Read the model definition and answer for the solid it produces. Units are mm, in the model's axes. Face numbers are marked on the shaded views. Coordinates: 2 decimals unless noted, no trailing zeros. Write each loop counter-clockwise with the first axis right and the second up, starting at its lowest first coordinate (ties: lowest second). Pieces come first, ordered by that corner, then holes.
(1) The part is cut by section D-D, the plane y = 71.5. Determine the outline of the cut face in (x, z).
(2) The part is cut by section A-A, the plane z = 6.5. Determine the outline of the cut face in (x, y), and give its area (3 significant figures).
(3) Straight lines are drawn through the part: line 1 along X through (y, z) = (116, 31.5); line 2 along Y through (x, z) = (4, 33.25); line 3 along X through (y, z) = (36, 23.5). For each, find the intervals that lie inside material, in ascending order.
(4) The part is cut by section B-B, the plane x = 58. Determine the outline of the cut face in (y, z).
(5) Given pin 1 (1.5 mm diameter, centred on x = 81.5, y = 110, fed in from +Z), flat-ended and moving along its own axis, determine where the tip first touches the part or whether it passes through.
(6) Determine the mould class of the marked faces 1, 2, 3 and 4 for opening direction X: pulls with the +X half, pulls with the -X half, needs draft (parallel to the pull), parting line crosses it, or undercut.
(7) The part is cut by section C-C, the plane x = 41. Determine the outline of the cut face in (y, z), and give its area (3 significant figures).
```python
from build123d import *

# Parameters (mm, degrees)
F0_W      = 88
F0_H      = 120
F1_DEPTH  = 3
F2_W      = 88
F2_H      = 120
F3_DEPTH  = 40
F5_DEPTH  = 3
F7_DEPTH  = 3
F8_R      = 0.5
F10_DEPTH = 20
F13_D     = 2.5
F13_DEPTH = 10
F13_TIP   = 0.7510757738
F15_DEPTH = 43
F17_DEPTH = 43
F18_W     = 10
F18_H     = 0.75
F19_DEPTH = 3
F21_D     = 2.5
F21_DEPTH = 25
F21_TIP   = 0.7510757738
F22_W     = 18
F22_H     = 3
F23_DEPTH = 3
F24_W     = 2
F24_H     = 12
F25_DEPTH = 3


with BuildPart() as f1:
    # F0 (on Top) → F1 (new body)
    with BuildSketch(Plane.XY):
        with Locations((44, 60)):
            Rectangle(F0_W, F0_H)
    extrude(amount=F1_DEPTH)

    # F2 (on face) → F3 (join)
    with BuildSketch(Plane.XY.offset(3)):
        with Locations((44, 60)):
            Rectangle(F2_W, F2_H)
        with BuildLine():
            ThreePointArc((3, 113.1715728753), (6.1213203436, 113.8786796564), (6.8284271247, 117))
            Line((6.8284271247, 117), (81.1715728753, 117))
            ThreePointArc((81.1715728753, 117), (81.8786796564, 113.8786796564), (85, 113.1715728753))
            Line((85, 113.1715728753), (85, 6.8284271247))
            ThreePointArc((85, 6.8284271247), (81.8786796564, 6.1213203436), (81.1715728753, 3))
            Line((81.1715728753, 3), (6.8284271247, 3))
            ThreePointArc((6.8284271247, 3), (6.1213203436, 6.1213203436), (3, 6.8284271247))
            Line((3, 6.8284271247), (3, 113.1715728753))
        make_face(mode=Mode.SUBTRACT)
    extrude(amount=F3_DEPTH)

    # F4 (on face) → F5 (cut, through all)
    with BuildSketch(Plane(origin=(0, 0, 0), x_dir=(0, -1, 0), z_dir=(-1, 0, 0))):
        with BuildLine():
            Line((-61.5, 38.8388347648), (-65.9194173824, 34.4194173824))
            ThreePointArc((-65.9194173824, 34.4194173824), (-61.5, 23.75), (-57.0805826176, 34.4194173824))
            Line((-57.0805826176, 34.4194173824), (-61.5, 38.8388347648))
        make_face()
        with BuildLine():
            Line((-39.0805826176, 34.4194173824), (-43.5, 38.8388347648))
            Line((-43.5, 38.8388347648), (-47.9194173824, 34.4194173824))
            ThreePointArc((-47.9194173824, 34.4194173824), (-43.5, 23.75), (-39.0805826176, 34.4194173824))
        make_face()
        with BuildLine():
            Line((-21.0805826176, 34.4194173824), (-25.5, 38.8388347648))
            Line((-25.5, 38.8388347648), (-29.9194173824, 34.4194173824))
            ThreePointArc((-29.9194173824, 34.4194173824), (-25.5, 23.75), (-21.0805826176, 34.4194173824))
        make_face()
    extrude(amount=-F5_DEPTH, mode=Mode.SUBTRACT)

    # F6 (on face) → F7 (cut, through all)
    with BuildSketch(Plane(origin=(0, 120, 0), x_dir=(-1, 0, 0), z_dir=(0, 1, 0))):
        with BuildLine():
            Line((-54.9344657888, 16.95), (-61.0655342112, 16.95))
            ThreePointArc((-61.0655342112, 16.95), (-58, 8), (-54.9344657888, 16.95))
        make_face()
    extrude(amount=-F7_DEPTH, mode=Mode.SUBTRACT)

    # F8
    f8_edges = [f1.edges().sort_by_distance(p)[0] for p in [
        (0, 60, 0),
        (44, 0, 0),
        (0, 0, 21.5),
        (0, 120, 21.5),
        (88, 0, 21.5),
        (88, 60, 0),
        (44, 120, 0),
        (88, 120, 21.5),
    ]]
    fillet(f8_edges, radius=F8_R)

    # F9 (on face) → F10 (join)
    with BuildSketch(Plane.XY.offset(3)):
        with BuildLine():
            Line((6.5, 84), (3, 84))
            Line((3, 84), (3, 74))
            Line((3, 74), (6.5, 74))
            ThreePointArc((6.5, 74), (11.5, 79), (6.5, 84))
        make_face()
        with BuildLine():
            Line((3, 105), (6.5, 105))
            ThreePointArc((6.5, 105), (10.0355339059, 106.4644660941), (11.5, 110))
            Line((11.5, 110), (11.5, 117))
            Line((11.5, 117), (6.8284271247, 117))
            ThreePointArc((6.8284271247, 117), (6.1213203436, 113.8786796564), (3, 113.1715728753))
            Line((3, 113.1715728753), (3, 105))
        make_face()
        with BuildLine():
            Line((81.1715728753, 117), (76.5, 117))
            Line((76.5, 117), (76.5, 110))
            ThreePointArc((76.5, 110), (77.9644660941, 106.4644660941), (81.5, 105))
            Line((81.5, 105), (85, 105))
            Line((85, 105), (85, 113.1715728753))
            ThreePointArc((85, 113.1715728753), (81.8786796564, 113.8786796564), (81.1715728753, 117))
        make_face()
        with BuildLine():
            Line((85, 74), (85, 84))
            Line((85, 84), (81.5, 84))
            ThreePointArc((81.5, 84), (76.5, 79), (81.5, 74))
            Line((81.5, 74), (85, 74))
        make_face()
    extrude(amount=F10_DEPTH)

    # F13
    with Locations(Plane.XY.offset(23)):
        with Locations((6.5, 110), (6.5, 79), (81.5, 79), (81.5, 110)):
            Hole(F13_D / 2, depth=F13_DEPTH)
            with Locations((0, 0, -(F13_DEPTH + F13_TIP / 2))):  # 118° drill point
                Cone(0, F13_D / 2, F13_TIP, mode=Mode.SUBTRACT)

    # F14 (on face) → F15 (cut, through all)
    with BuildSketch(Plane.XZ.offset(-74)):
        Polygon((76.5, 3), (85, 3), (85, 9), (76.5, 21.1392580573), align=None)
    extrude(amount=-F15_DEPTH, mode=Mode.SUBTRACT)

    # F16 (on face) → F17 (cut, through all)
    with BuildSketch(Plane.XZ.offset(-74)):
        Polygon((3, 9), (3, 3), (11.5, 3), (11.5, 21.1392580573), align=None)
    extrude(amount=-F17_DEPTH, mode=Mode.SUBTRACT)

    # F18 (on face) → F19 (cut, through all)
    with BuildSketch(Plane.XY.offset(3)):
        with Locations((80, 7.875)):
            Rectangle(F18_W, F18_H)
        with Locations((80, 15.875)):
            Rectangle(F18_W, F18_H)
        with Locations((80, 108.625)):
            Rectangle(F18_W, F18_H)
        with Locations((80, 116.625)):
            Rectangle(F18_W, F18_H)
    extrude(amount=-F19_DEPTH, mode=Mode.SUBTRACT)

    # F21
    with Locations(Plane.XY.offset(43)):
        with Locations((4, 116), (4, 4), (84, 4), (84, 116)):
            Hole(F21_D / 2, depth=F21_DEPTH)
            with Locations((0, 0, -(F21_DEPTH + F21_TIP / 2))):  # 118° drill point
                Cone(0, F21_D / 2, F21_TIP, mode=Mode.SUBTRACT)

    # F22 (on face) → F23 (cut, through all)
    with BuildSketch(Plane(origin=(0, 0, 0), x_dir=(0, -1, 0), z_dir=(-1, 0, 0))):
        with Locations((-94.25, 31.5)):
            Rectangle(F22_W, F22_H)
    extrude(amount=-F23_DEPTH, mode=Mode.SUBTRACT)

    # F24 (on face) → F25 (cut, through all)
    with BuildSketch(Plane.YZ.offset(88)):
        with Locations((87.5, 16)):
            Rectangle(F24_W, F24_H)
        with Locations((91, 16)):
            Rectangle(F24_W, F24_H)
        with Locations((94.5, 16)):
            Rectangle(F24_W, F24_H)
        with Locations((98, 16)):
            Rectangle(F24_W, F24_H)
        with Locations((101.5, 16)):
            Rectangle(F24_W, F24_H)
    extrude(amount=-F25_DEPTH, mode=Mode.SUBTRACT)


solid = f1.part
```
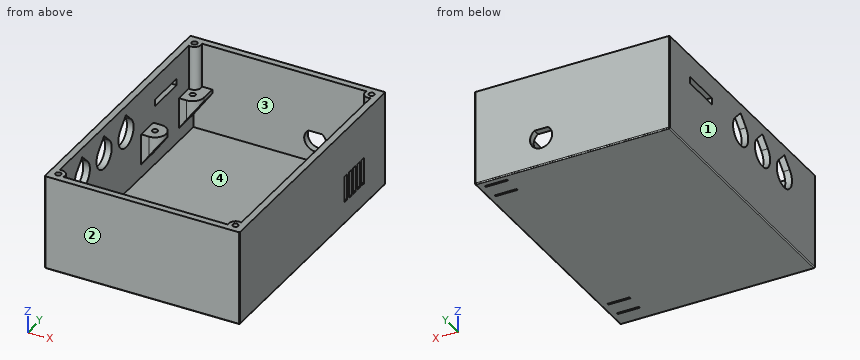
Computed:
1. outline: (0, 0.5) arc R0.5 ccw to (0.5, 0) - (87.5, 0) arc R0.5 ccw to (88, 0.5) - (88, 43) - (85, 43) - (85, 3) - (3, 3) - (3, 43) - (0, 43) - close
2. outline: (0, 0.5) arc R0.5 ccw to (0.5, 0) - (87.5, 0) arc R0.5 ccw to (88, 0.5) - (88, 119.5) arc R0.5 ccw to (87.5, 120) - (0.5, 120) arc R0.5 ccw to (0, 119.5) - close; hole (3, 6.83) arc R3 cw to (6.83, 3) - (81.17, 3) arc R3 cw to (85, 6.83) - (85, 117) - (3, 117) - close
2. area: 1,240 mm2
3. line 1: x = 0 to 2.75, 5.25 to 7, 81 to 82.75, 85.25 to 88
3. line 2: y = 0 to 2.75, 5.25 to 7, 113 to 114.75, 117.25 to 120
3. line 3: x = 0 to 3, 85 to 88
4. outline: (0, 0.5) arc R0.5 ccw to (0.5, 0) - (119.5, 0) arc R0.5 ccw to (120, 0.5) - (120, 8) - (117, 8) - (117, 3) - (3, 3) - (3, 43) - (0, 43) - close; (117, 16.95) - (120, 16.95) - (120, 43) - (117, 43) - close
5. pin 1: stops at z = 3
6. face 1: pulls with the -X half
6. face 2: needs draft
6. face 3: undercut
6. face 4: undercut
7. outline: (0, 0.5) arc R0.5 ccw to (0.5, 0) - (119.5, 0) arc R0.5 ccw to (120, 0.5) - (120, 43) - (117, 43) - (117, 3) - (3, 3) - (3, 43) - (0, 43) - close
7. area: 600 mm2
